Design review of the part shown in the three views and the two pictorial views. Dimensions are in mm from the part's minimum x, y and z. Coordinates: 2 decimals unless noted, no trailing zeros. Loops run counter-clockwise (first coordinate to the right, second up) from the corner with the lowest first, then second, coordinate; pieces in that order, holes last. Notation, with made-up numbers: (-20, 30.25) -> (22, 30.25) arc R5 ccw to (22, 36.25) -> close; hole circle Ø3 at (84, 64.25). An arc over 180 degrees is marked (long way). Answer in a Markdown table with one row per item.
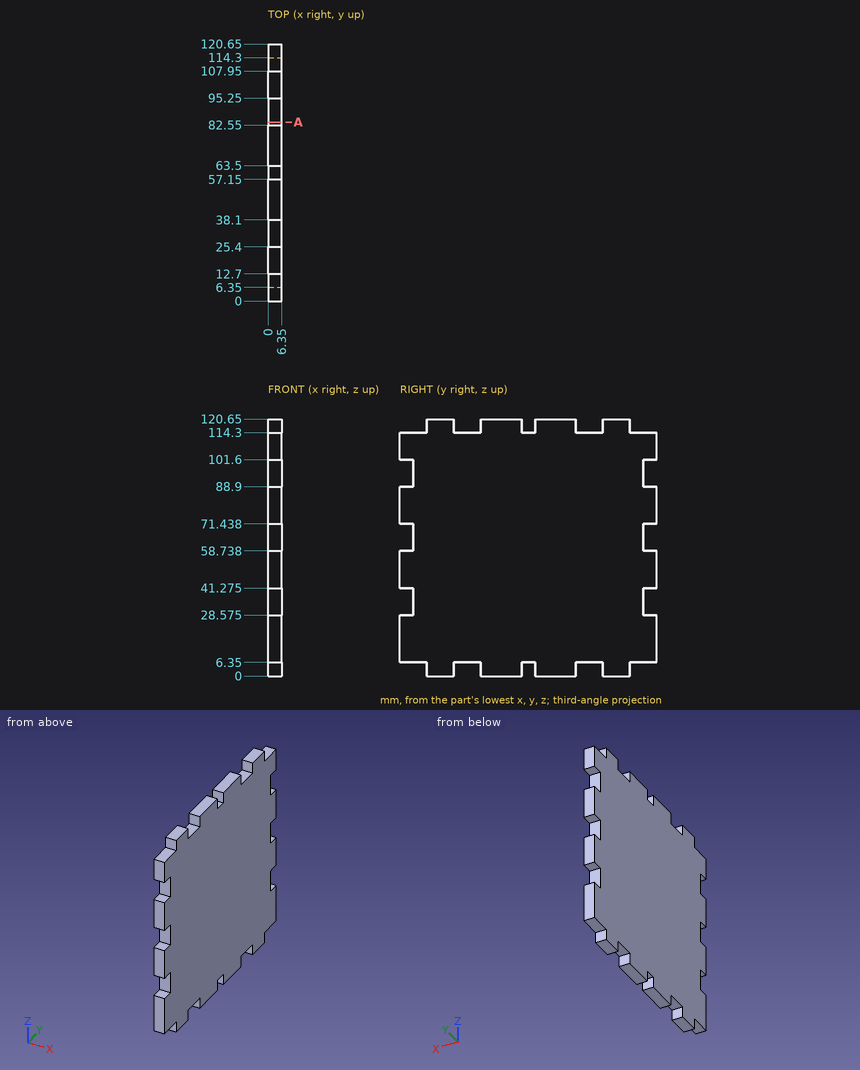
(1) For pin 1 (4 mm diameter, centred on y = 26.5, z = 97.5, fed in from -X); pin 2 (1.9 mm diameter, centred on x = 4.5, z = 118, fed in from -Y); pin 3 (1.9 mm diameter, centred on x = 3, z = 68, fed in from -Y); pin 4 (3 mm diameter, centred on x = 3, z = 117.5, fed in from +Y), all flat-tipped, find the tip position at first contact; note any pin that passes through.
Evaluation:
| item | result |
|---|---|
| pin 1 | stops at x = 0 |
| pin 2 | stops at y = 12.7 |
| pin 3 | stops at y = 6.35 |
| pin 4 | stops at y = 107.95 |
(2) Take a section at A-A on y = 84. Give the boundary of the cut face in (x, z).
Evaluation:
| item | result |
|---|---|
| outline | (0, 6.35) -> (6.35, 6.35) -> (6.35, 114.3) -> (0, 114.3) -> close |
(3) To check wall thickness, follow probe 1 along Y at (x, z) = (2, 6); probe 2 along Z at (x, y) = (4.75, 34.5). State the ranges of each line that lie inside material, in increasing order.
Evaluation:
| item | result |
|---|---|
| probe 1 | y = 12.7 to 25.4, 38.1 to 57.15, 63.5 to 82.55, 95.25 to 107.95 |
| probe 2 | z = 6.35 to 114.3 |
